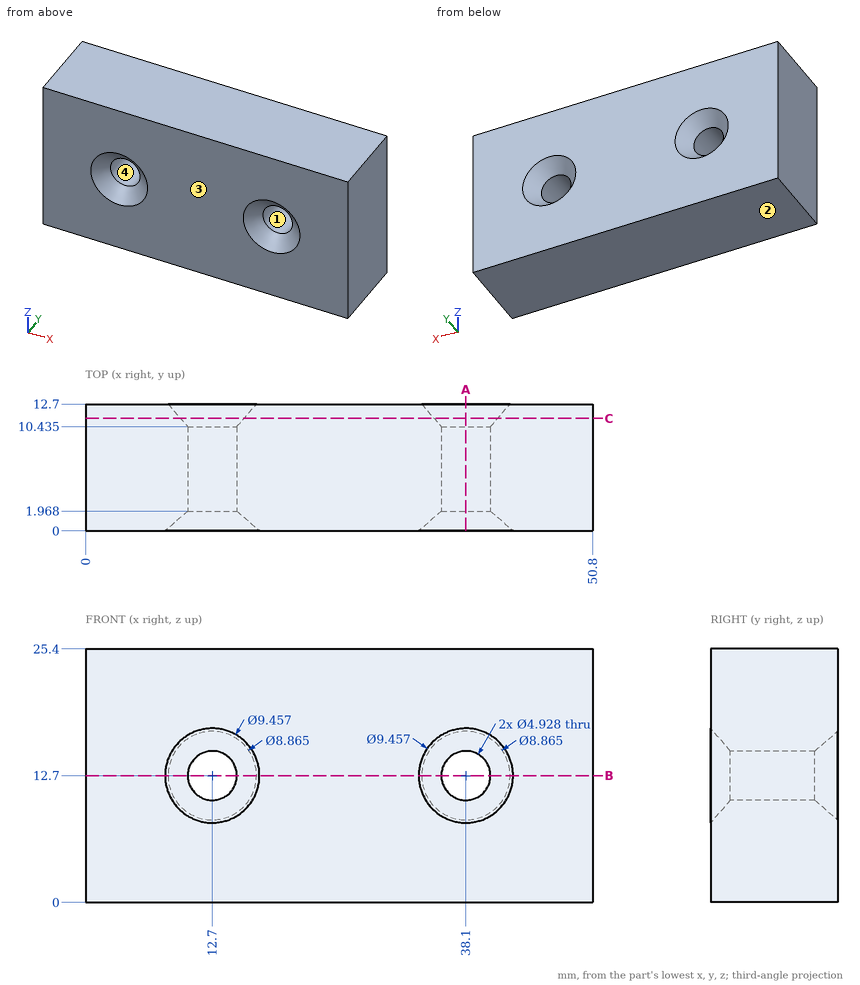
Study the drawing (mm; zero at the part's minimum x, y, z) and answer. Coordinates: 2 decimals unless noted, no trailing zeros. Order: outer loops, then holes, each group sorted by start corner. A loop starts at its lowest first (then second) coordinate and runs counter-clockwise, first axis right, second up. Notation, with made-up numbers: M -5.5,-19 L 13.5,-19 A15 ccw 13.5,10 Z; hole C -17.75,83.25 d7. An arc over 180 degrees is marked long. Answer as a JSON object with one key per item and string values. Group by question number.
1. A flat-ended cylindrical pin translates along its axis: P1, Ø5.5, axis at x = 12.7, z = 12.7, coming from the +Y side (1 decimal). Find the tip coordinate at first contact, or state that the pin passes through.
2. Section B-B on z = 12.7 is taken. Write down the section's boundary in (x, y) (1 decimal), then the cut area to 3 significant figures.
3. Section C-C on y = 11.25 is taken. Write down the section's boundary in (x, z), then the cut area to 3 significant figures.
4. Determine the mould class of the marked faces 1, 2, 3 and 4 for opening direction Z: released by +Z, released by -Z, zero draft, split by the parting line, or undercut.
5. Section A-A on x = 38.1 is taken. Write down the section's boundary in (y, z) (1 decimal), then the cut area to 3 significant figures.
6. Straight lines are drawn through the part: line 1 (X direction, y = 6, z = 12.7); line 2 (Z direction, x = 12.7, y = 4.75); line 3 (X direction, y = 6.5, z = 13.75). For each, find the intervals that lie inside material, in ascending order.
Values follow:
{
 "1": {"P1": "y = 10.8"},
 "2": {"outline": "M 0,0 L 8,0 L 10.2,2 L 10.2,10.4 L 8.3,12.7 L 0,12.7 Z; M 15.2,2 L 17.4,0 L 33.4,0 L 35.6,2 L 35.6,10.4 L 33.7,12.7 L 17.1,12.7 L 15.2,10.4 Z; M 40.6,2 L 42.8,0 L 50.8,0 L 50.8,12.7 L 42.5,12.7 L 40.6,10.4 Z", "area": "502 mm2"},
 "3": {"outline": "M 0,0 L 50.8,0 L 50.8,25.4 L 0,25.4 Z; hole C 12.7,12.7 d6.34; hole C 38.1,12.7 d6.34", "area": "1,230 mm2"},
 "4": {"face 1": "undercut", "face 2": "released by -Z", "face 3": "zero draft", "face 4": "undercut"},
 "5": {"outline": "M 0,0 L 12.7,0 L 12.7,8.3 L 10.4,10.2 L 2,10.2 L 0,8 Z; M 0,17.4 L 2,15.2 L 10.4,15.2 L 12.7,17.1 L 12.7,25.4 L 0,25.4 Z", "area": "251 mm2"},
 "6": {"line 1": "0 to 10.24, 15.16 to 35.64, 40.56 to 50.8", "line 2": "0 to 10.24, 15.16 to 25.4", "line 3": "0 to 10.47, 14.93 to 35.87, 40.33 to 50.8"}
}
